Source: CAD feature listing. Evaluate the final solid. Frame: model axes, mm. A direction names the side the tool comes from. Coordinates: 2 decimals unless noted, no trailing zeros. Order: outer loops, then holes, each group sorted by start corner. A loop starts at its lowest first (then second) coordinate and runs counter-clockwise, first axis right, second up.
Item 1: Section B-B on x = -16.5. Return the cut outline in (y, z).
Item 2: Section A-A on z = 11. Return the cut outline in (x, y), then the cut area to 3 significant figures.
Item 3: Ray query, line 1 (Z direction, x = -36.5, y = 75.5); line 2 (X direction, y = 64, z = 11.5); line 3 (Y direction, x = -54, z = 27.5). Return the intervals inside material, ascending.
Item 4: Section D-D on z = 64.5. Return the cut outline in (x, y), then the cut area to 3 significant figures.
Item 5: Contact query for flat-ended pins moving along their axis: P1, Ø10, axis at x = -50, z = 27.5, coming from the +Y side; P2, Ø8, axis at x = -68, y = 29, coming from the +Z side; P3, Ø8, axis at x = -23.5, z = 34.5, coming from the -Y side. Output: stop coordinate, or through.
Item 6: Section C-C on y = 62.5. Return the cut outline in (x, z), then the cut area to 3 significant figures.
Item 7: Reachability of faces 1 (the flat face through (-51, 51, 0)), 2 (the cylindrical face through (-60.05, 58.744, 63.322)) from +Z, -Z, +X, -X, +Y, -Y: full face, straight path, thin tool, end or side. Return the list, or none.
from build123d import *

# Parameters (mm, degrees)
F1_DEPTH = 76.2
F2_DEPTH = 50.8


with BuildPart() as f1:
    # F0 (on Top) → F1 (new body)
    with BuildSketch(Plane.XY):
        with BuildLine():
            Line((0, 84.0056133164), (0, 100.8445028668))
            ThreePointArc((0, 100.8445028668), (-71.3078318225, 71.3078318225), (-100.8445028668, 0))
            Line((-100.8445028668, 0), (-84.0056133164, 0))
            ThreePointArc((-84.0056133164, 0), (-59.4009388338, 59.4009388338), (0, 84.0056133164))
        make_face()
    extrude(amount=F1_DEPTH)

    # F0 (on Top) → F2 (join)
    with BuildSketch(Plane.XY):
        with BuildLine():
            Line((0, 52.9438169528), (0, 84.0056133164))
            ThreePointArc((0, 84.0056133164), (-59.4009388338, 59.4009388338), (-84.0056133164, 0))
            Line((-84.0056133164, 0), (-52.9438169528, 0))
            ThreePointArc((-52.9438169528, 0), (-37.4369319892, 37.4369319892), (0, 52.9438169528))
        make_face()
    extrude(amount=F2_DEPTH)


solid = f1.part
Answer list:
1. outline: (50.31, 0) - (99.49, 0) - (99.49, 76.2) - (82.37, 76.2) - (82.37, 50.8) - (50.31, 50.8) - close
2. outline: (-100.84, 0) - (-52.94, 0) arc R52.94 cw to (0, 52.94) - (0, 100.84) arc R100.84 ccw to start
2. area: 5,790 mm2
3. line 1: z = 0 to 50.8
3. line 2: x = -77.93 to 0
3. line 3: y = 0 to 85.17
4. outline: (-100.84, 0) - (-84.01, 0) arc R84.01 cw to (0, 84.01) - (0, 100.84) arc R100.84 ccw to start
4. area: 2,440 mm2
5. P1: stops at y = 90.25
5. P2: stops at z = 50.8
5. P3: stops at y = 45.24
6. outline: (-79.14, 0) - (0, 0) - (0, 50.8) - (-56.13, 50.8) - (-56.13, 76.2) - (-79.14, 76.2) - close
6. area: 4,600 mm2
7. face 1: -Z, +X, -X, +Y, -Y
7. face 2: +Z, +X, -Y
